The listing builds one solid part. Answer for the finished solid, in the listing's coordinates (mm). A direction names the side the tool comes from. Give positions to 0.01 mm unless a question says otherwise; leave off trailing zeros. Write each loop counter-clockwise with the first axis right and the second up, starting at its lowest first coordinate (ties: lowest second). Pieces come first, ordered by that corner, then holes. Notation, with made-up numbers: M 24,71 L 66,71 A13 cw 66,85 Z; hole C 19.25,26 d11. An arc over 180 degrees is marked long. Answer as a JSON object with one key per item and string values.
```python
from build123d import *

# Parameters (mm, degrees)
SKETCH1_W           = 40.259
SKETCH1_H           = 25.4
SKETCH1_R           = 1.905
BOSS_EXTRUDE1_DEPTH = 9.525
BOSS_EXTRUDE2_DEPTH = 127
SKETCH3_R           = 1.905
BOSS_EXTRUDE3_DEPTH = 9.525
FILLET2_R           = 6.35
FILLET3_R           = 3.175
CUT_EXTRUDE1_REACH  = 153.604
SKETCH4_W           = 40.259
SKETCH4_H           = 3.175
FILLET4_R           = 9.525
FILLET6_R           = 6.35


with BuildPart() as part:
    # Sketch1 → Boss-Extrude1 (new body)
    with BuildSketch(Plane.XY):
        with Locations((-11.6205, 12.7)):
            Rectangle(SKETCH1_W, SKETCH1_H)
        with Locations(Location((-22.225, 9.525, 0), (0, 0, 180))):
            Circle(SKETCH1_R, mode=Mode.SUBTRACT)
        with Locations(Location((-25.4, 19.05, 0), (0, 0, 180))):
            Circle(SKETCH1_R, mode=Mode.SUBTRACT)
    extrude(amount=BOSS_EXTRUDE1_DEPTH)

    # Sketch2 → Boss-Extrude2 (add)
    with BuildSketch(Plane.XY.offset(9.525)):
        Polygon((-19.05, 25.4), (-9.525, 0), (8.509, 0), (8.509, 25.4), align=None)
    extrude(amount=BOSS_EXTRUDE2_DEPTH)

    # Sketch3 → Boss-Extrude3 (add)
    with BuildSketch(Plane.XY.offset(136.525)):
        Polygon((8.509, 25.4), (-19.05, 25.4), (-31.75, 25.4), (-31.75, 0), (-9.525, 0), (8.509, 0), align=None)
        with Locations(Location((-25.4, 19.05, 0), (0, 0, 180))):
            Circle(SKETCH3_R, mode=Mode.SUBTRACT)
        with Locations(Location((-22.225, 9.525, 0), (0, 0, 180))):
            Circle(SKETCH3_R, mode=Mode.SUBTRACT)
    extrude(amount=BOSS_EXTRUDE3_DEPTH)

    # Fillet2
    fillet2_edges = [part.edges().sort_by_distance(p)[0] for p in [
        (-31.75, 25.4, 4.7625),
        (8.509, 25.4, 73.025),
        (-31.75, 25.4, 141.2875),
    ]]
    fillet(fillet2_edges, radius=FILLET2_R)

    # Fillet3
    fillet3_edges = [part.edges().sort_by_distance(p)[0] for p in [
        (-19.05, 25.4, 73.025),
    ]]
    fillet(fillet3_edges, radius=FILLET3_R)

    # Cut-Extrude1: up to this face of the body (flat: up to its plane)
    cut_extrude1_end = Plane(part.part.faces().sort_by_distance((-11.337539772, 12.464426548, 0))[0])
    # Sketch4 → Cut-Extrude1 (cut, up to the picked face)
    with BuildSketch(Plane.XY.offset(146.05), mode=Mode.PRIVATE) as cut_extrude1_sk1:
        with Locations((-11.6205, 1.5875)):
            Rectangle(SKETCH4_W, SKETCH4_H)
    cut_extrude1_tool1 = split(extrude(cut_extrude1_sk1.sketch, amount=-CUT_EXTRUDE1_REACH, mode=Mode.PRIVATE), bisect_by=cut_extrude1_end, keep=Keep.BOTH, mode=Mode.PRIVATE)
    add(cut_extrude1_tool1.solids().sort_by(Axis((-11.6205, 1.5875, 146.05), (0, 0, -1)))[0], mode=Mode.SUBTRACT)

    # Fillet4
    fillet4_edges = [part.edges().sort_by_distance(p)[0] for p in [
        (-31.75, 3.175, 141.2875),
        (-31.75, 3.175, 4.7625),
    ]]
    fillet(fillet4_edges, radius=FILLET4_R)

    # Fillet6
    fillet6_edges = [part.edges().sort_by_distance(p)[0] for p in [
        (8.509, 3.175, 73.025),
    ]]
    fillet(fillet6_edges, radius=FILLET6_R)


solid = part.part
```
1. Consider line 1 along X through (y, z) = (19.05, 6) (3 decimals); line 2 along Z through (x, y) = (-27, 13) (3 decimals); line 3 along Y through (x, z) = (-25.4, 2) (3 decimals). Determine where each line is inside the solid, lowest interval first.
Verdict:
{"line 1": "x = -31.75 to -27.305, -23.495 to 8.509", "line 2": "z = 0 to 9.525, 136.525 to 146.05", "line 3": "y = 3.72 to 17.145, 20.955 to 25.4"}
2. A cutting plane is placed at B-B, the plane x = 5. Give the vertices of the cut face in (y, z), plus the area to 3 significant figures.
Verdict:
{"outline": "M 3.85,0 L 24.73,0 L 24.73,146.05 L 3.85,146.05 Z", "area": "3,050 mm2"}
3. For faces 1 (the flat face through (-14.126, 12.268, 72.136)), 2 (the cylindrical face through (-17.05, 24.07, 73.91)), 3 (the cylindrical face through (-24, 17.76, 141.22)), determine the directions among +Z, -Z, +X, -X, +Y, -Y from which every point of the face is accessible in a straight line to the end or side of a thin tool.
Verdict:
{"face 1": "-X, -Y", "face 2": "-X", "face 3": "+Z, -Z"}
4. Flat-ended cylindrical pins translate along their axes: pin 1 (12 mm diameter, centred on x = 3.5, z = 22.5, fed in from +Y); pin 2 (10 mm diameter, centred on y = 13.5, z = 25, fed in from -X); pin 3 (2 mm diameter, centred on y = 8.5, z = 33.5, fed in from -X); pin 4 (4 mm diameter, centred on y = 21.5, z = 115.5, fed in from -X). Find the tip coordinate at first contact, or state that the pin passes through.
Verdict:
{"pin 1": "stops at y = 25.4", "pin 2": "stops at x = -16.46", "pin 3": "stops at x = -13.09", "pin 4": "stops at x = -17.64"}
5. The mould has two halves that part along Y. Classify faces 4 (the flat face through (-31.75, 16, 141)), 5 (the flat face through (-7, 3.175, 74)), 6 (the cylindrical face through (-20.32, 9.44, 4.7)): released by +Y, released by -Y, zero draft, split by the parting line, or undercut.
Verdict:
{"face 4": "zero draft", "face 5": "released by -Y", "face 6": "undercut"}
6. A cutting plane is placed at A-A, the plane z = 22. Give the vertices of the cut face in (x, y) (3 decimals), plus the area to 3 significant figures.
Verdict:
{"outline": "M -17.441,21.11 L -10.716,3.175 L 2.159,3.175 A6.35 ccw 8.509,9.525 L 8.509,19.05 A6.35 ccw 2.159,25.4 L -14.468,25.4 A3.175 ccw Z", "area": "498 mm2"}
